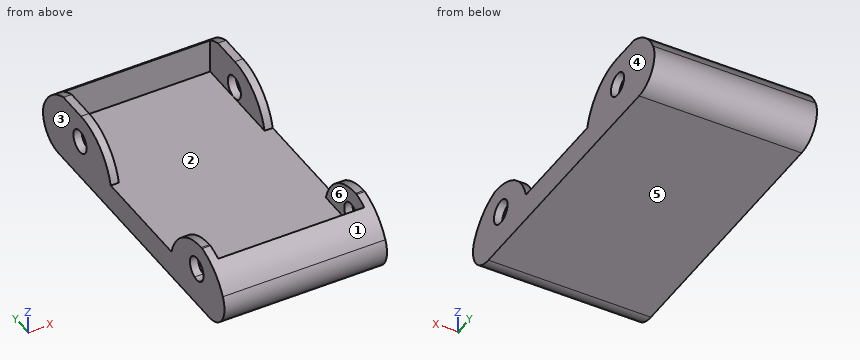
Autodesk Inventor part; units mm, degrees
ref_plane "YZ Plane" through (0, 0, 0) normal (1, 0, 0) x (0, 1, 0)
ref_plane "XZ Plane" through (0, 0, 0) normal (0, 1, 0) x (-1, 0, 0)
ref_plane "XY Plane" through (0, 0, 0) normal (0, 0, 1) x (1, 0, 0)
sketch "Sketch1" plane through (0, 0, 0) normal (0, 0, 1) x (1, 0, 0)
  line L0 (-7.6725, 9.18) -> (144.7275, 9.18)
  line L1 (144.7275, 9.18) -> (144.7275, -295.62)
  line L2 (144.7275, -295.62) -> (-7.6725, -295.62)
  line L3 (-7.6725, -295.62) -> (-7.6725, 9.18)
  point P0 (0, 0)
  dimension "d0" = 152.4
  dimension "d1" = 304.8
extrude "Extrusion1" add sketch "Sketch1" along normal blind 25.4
sketch "Sketch2" plane through (0, 0, 25.4) normal (0, 0, 1) x (1, 0, 0)
  line L0 (144.7275, 9.18) -> (-7.6725, 9.18)
  line L1 (-7.6725, 9.18) -> (-7.6725, -26.9908)
  line L2 (-7.6725, 9.18) -> (-7.6725, -295.62)
  line L3 (144.7275, -295.62) -> (144.7275, 9.18)
  line L4 (144.7275, 9.18) -> (144.7275, -26.9908)
  line L5 (144.7275, -26.9908) -> (-7.6725, -26.9908)
  line L6 (-7.6725, 9.18) -> (144.7275, 9.18)
  point P0 (0, 0)
extrude "Extrusion2" add sketch "Sketch2" along normal blind 38.1
fillet "Fillet1" radius 50.8 1 edges at (68.5275, 9.18, 63.5)
sketch "Sketch3" plane through (0, 0, 25.4) normal (0, 0, 1) x (1, 0, 0)
  line L0 (-7.6725, -26.9908) -> (-7.6725, -295.62)
  line L1 (-7.6725, -26.9908) -> (-7.6725, -104.161)
  line L2 (0, -104.161) -> (0, -26.9908)
  line L3 (0, -26.9908) -> (-7.6725, -26.9908)
  line L4 (0, -104.161) -> (-7.6725, -104.161)
  line L5 (144.7275, -26.9908) -> (-7.6725, -26.9908)
  line L6 (144.7275, -26.9908) -> (137.0567, -26.9908)
  line L7 (137.0567, -26.9908) -> (137.0567, -104.161)
  line L8 (137.0567, -104.161) -> (144.7275, -104.161)
  line L9 (144.7275, 9.18) -> (144.7275, -295.62)
  line L10 (144.7275, -26.9908) -> (144.7275, -104.161)
  point P0 (0, 0)
  dimension "d7" = 7.6708
extrude "Extrusion3" add sketch "Sketch3" along normal blind 38.1 contours L9 L8 L7 L5
sketch "Sketch4" plane through (0, 0, 25.4) normal (0, 0, 1) x (1, 0, 0)
  line L0 (-7.6725, -26.9908) -> (-7.6725, 9.18)
  line L1 (-7.6725, -26.9908) -> (0, -26.9908)
  line L2 (137.0567, -26.9908) -> (-7.6725, -26.9908)
  line L3 (-7.6725, -295.62) -> (-7.6725, 9.18)
  line L4 (0, -104.9824) -> (-7.6725, -104.9824)
  line L5 (-7.6725, -26.9908) -> (-7.6725, -104.9824)
  line L6 (0, -104.9824) -> (0, -26.9908)
  point P0 (0, 0)
extrude "Extrusion4" add sketch "Sketch4" along normal blind 38.1
fillet "Fillet2" radius 50.8 1 edges at (-3.8363, -104.9824, 63.5)
fillet "Fillet3" radius 50.8 1 edges at (140.8921, -104.161, 63.5)
sketch "Sketch5" plane through (137.0567, -26.9908, 25.4) normal (0, -1, 0) x (1, 0, 0)
  line L0 (-137.0567, 38.1) -> (0, 38.1)
  line L1 (-137.0567, 38.1) -> (-137.0567, 0)
  line L2 (-137.0567, 38.1) -> (-137.0567, 0)
  line L3 (0, 0) -> (-137.0567, 0)
  line L4 (-137.0567, 0) -> (0, 0)
  line L5 (0, 0) -> (0, 38.1)
  line L6 (0, 0) -> (0, 38.1)
  line L7 (0, 38.1) -> (-137.0567, 38.1)
  point P0 (-137.0567, -25.4)
extrude "Extrusion5" cut sketch "Sketch5" against normal blind 12.7
sketch "Sketch6" plane through (0, 0, 25.4) normal (0, 0, 1) x (1, 0, 0)
  line L0 (-7.6725, -295.62) -> (-7.6725, 9.18)
  line L1 (144.7275, -295.62) -> (-7.6725, -295.62)
  line L2 (-7.6725, -295.62) -> (-7.6725, -256.2446)
  line L3 (144.7275, -295.62) -> (144.7275, -256.2446)
  line L4 (144.7275, -295.62) -> (144.7275, -104.161)
  line L5 (-7.6725, -256.2446) -> (144.7275, -256.2446)
  point P0 (0, 0)
extrude "Extrusion6" add sketch "Sketch6" along normal blind 38.1
fillet "Fillet4" radius 50.8 1 edges at (68.5275, -295.62, 63.5)
sketch "Sketch7" plane through (0, 0, 25.4) normal (0, 0, 1) x (1, 0, 0)
  line L0 (137.676, -256.2446) -> (144.7275, -256.2446)
  line L1 (-7.6725, -295.62) -> (-7.6725, 9.18)
  line L2 (-7.6725, -256.2446) -> (144.7275, -256.2446)
  line L3 (-7.6725, -256.2446) -> (-7.6725, -205.4446)
  line L4 (-7.6725, -205.4446) -> (0, -205.4446)
  line L5 (0, -205.4446) -> (0, -256.2446)
  point P0 (0, 0)
  dimension "d20" = 50.8
extrude "Extrusion7" add sketch "Sketch7" along normal blind 38.1
sketch "Sketch8" plane through (0, 0, 25.4) normal (0, 0, 1) x (1, 0, 0)
  line L0 (0, -256.2446) -> (144.7275, -256.2446)
  line L1 (144.7275, -256.2446) -> (144.7275, -205.4446)
  line L2 (144.7275, -256.2446) -> (144.7275, -104.161)
  line L3 (144.7275, -205.4446) -> (137.0567, -205.4446)
  line L4 (137.0567, -205.4446) -> (137.0567, -256.2446)
  line L5 (137.0567, -256.2446) -> (144.7275, -256.2446)
  point P0 (0, 0)
  dimension "d23" = 50.8
  dimension "d24" = 7.6708
extrude "Extrusion8" add sketch "Sketch8" along normal blind 38.1
fillet "Fillet5" radius 50.8 2 edges at (-3.8363, -205.4446, 63.5) (140.8921, -205.4446, 63.5)
sketch "Sketch9" plane through (0, -256.2446, 63.5) normal (0, 1, 0) x (1, 0, 0)
  line L0 (0, 38.1) -> (137.0567, 38.1)
  line L1 (137.0567, 38.1) -> (0, 38.1)
  line L2 (0, 38.1) -> (0, 0)
  line L3 (0, 38.1) -> (0, 0)
  line L4 (137.0567, 0) -> (0, 0)
  line L5 (0, 0) -> (137.0567, 0)
  line L6 (137.0567, 0) -> (137.0567, 38.1)
  point P0 (0, 63.5)
extrude "Extrusion9" cut sketch "Sketch9" against normal blind 12.7
sketch "Sketch10" plane through (144.7275, -295.62, 0) normal (1, 0, 0) x (0, 0, -1)
  point P0 (0, 295.62)
fillet "Fillet6" radius 25.4 1 edges at (68.5275, -295.62, 0)
fillet "Fillet7" radius 25.4 1 edges at (68.5275, 9.18, 0)
sketch "Sketch21" plane through (0, 0, 25.4) normal (0, 0, 1) x (1, 0, 0)
  point P0 (0, 0)
sketch "Sketch22" plane through (0, 0, 25.4) normal (0, 0, 1) x (1, 0, 0)
  point P0 (0, 0)
sketch "Sketch23" plane through (0, -55.7956, 63.5) normal (1, 0, 0) x (0, 0, -1)
  point P0 (63.5, 55.7956)
sketch "Sketch24" plane through (0, -55.7956, 63.5) normal (1, 0, 0) x (0, 0, -1)
  circle A0 centre (27.2379, 1.6041) radius 10.8621
  line L0 (38.1, -49.1869) -> (38.1, 41.5047)
  point P0 (63.5, 55.7956)
extrude "Extrusion18" cut sketch "Sketch24" against normal blind 25.4
sketch "Sketch25" plane through (137.0567, -54.9742, 63.5) normal (-1, 0, 0) x (0, 0, 1)
  circle A0 centre (-27.2379, 0.7827) radius 10.8621
  circle A1 centre (-27.2379, 0.7827) radius 10.8621
  point P0 (-63.5, 54.9742)
extrude "Extrusion19" cut sketch "Sketch25" against normal blind 25.4
sketch "Sketch26" plane through (137.0567, -268.9446, 25.4) normal (-1, 0, 0) x (0, 0, 1)
  circle A0 centre (10.6882, 21.8663) radius 11.2364
  point P0 (-25.4, 268.9446)
extrude "Extrusion20" cut sketch "Sketch26" against normal blind 25.4
sketch "Sketch27" plane through (0, -268.9446, 25.4) normal (1, 0, 0) x (0, 0, -1)
  arc A0 (0, 25.3331) -> (0, 18.3996) centre (-10.6882, 21.8663) ccw
  circle A1 centre (-10.6882, 21.8663) radius 11.2364
  point P0 (25.4, 268.9446)
extrude "Extrusion21" cut sketch "Sketch27" against normal blind 25.4
properties part number "chasis for robot car"
Check sheet for the modelled part. Datum: model origin and axes. Units: mm. Face numbers are marked on the shaded views. A direction names the side the tool comes from. Give positions to 0.01 mm unless a question says otherwise; leave off trailing zeros. Write each loop counter-clockwise with the first axis right and the second up, starting at its lowest first coordinate (ties: lowest second). Pieces come first, ordered by that corner, then holes. Notation, with made-up numbers: (-4, -9) -> (17, -9) arc R11 cw to (17, -2) -> close; hole circle Ø7 at (60, 5). An arc over 180 degrees is marked (long way). One line per item, written item: value. Start each with the question number.
Item 1: Draft check along X on the marked faces 3, 4, 5 and 6. Enter one of: +X half, -X half, draft (parallel to the pull), parting line (faces both ways), or undercut.
Item 2: Tool access check on the marked faces 1 and 2. Record the directions out of +Z, -Z, +X, -X, +Y, -Y that give a thin tool (end or side, any length) a straight path to the whole face; none if there is none.
Item 3: Section check B-B on y = -261.5. Record the cut outline in (x, z).
Item 4: Section check C-C on z = 28.5. State how many separate pieces and enclosed holes the cut face has, then the cut area to 3 significant figures.
Item 5: Material ranges on probe 1 along Y at (x, z) = (119, 24); probe 2 along Z at (x, y) = (49, -21.5); probe 3 along Y at (x, z) = (59.5, 30), recorded low to high. Write a range as from..to.
Item 6: Gauge pin test, flat ends, axial feed: pin 1 (1.5 mm diameter, centred on x = 95, y = -99.5, fed in from +Z); pin 2 (1 mm diameter, centred on x = 93, z = 34, fed in from -Y); pin 3 (1.5 mm diameter, centred on x = 46, z = 46.5, fed in from -Y). Record the tip position at first contact, or that the pin passes through.
Item 7: Section check A-A on z = 53.5. Record the cut outline in (x, y), then the cut area to 3 significant figures.
Item 8: Section check D-D on y = -75.5. Record the cut outline in (x, z).
Results list:
1. face 3: -X half
1. face 4: +X half
1. face 5: draft
1. face 6: undercut
2. face 1: +Z, +X, -X, -Y
2. face 2: +Z
3. outline: (-7.67, 0) -> (144.73, 0) -> (144.73, 61.98) -> (137.06, 61.98) -> (137.06, 25.4) -> (0, 25.4) -> (0, 61.98) -> (-7.67, 61.98) -> close
4. separate pieces: 6
4. enclosed holes: 0
4. area: 8,670 mm²
5. probe 1: -292.88..6.85
5. probe 2: 0..25.4
5. probe 3: -292.5..-268.94, -14.29..6.47
6. pin 1: z = 25.4
6. pin 2: y = -291.59
6. pin 3: y = -284.48
7. outline: (-7.67, -276.77) -> (144.73, -276.77) -> (144.73, -224.37) -> (137.06, -224.37) -> (137.06, -268.94) -> (0, -268.94) -> (0, -224.37) -> (-7.67, -224.37) -> close; (-7.67, -86.06) -> (0, -86.06) -> (0, -14.29) -> (137.06, -14.29) -> (137.06, -85.24) -> (144.73, -85.24) -> (144.73, -8.65) -> (-7.67, -8.65) -> close
7. area: 3,830 mm²
8. outline: (-7.67, 0) -> (144.73, 0) -> (144.73, 59.17) -> (137.06, 59.17) -> (137.06, 25.4) -> (0, 25.4) -> (0, 59.52) -> (-7.67, 59.52) -> close
